Read the model definition and answer for the solid it produces. Units are mm, in the model's axes. Face numbers are marked on the shaded views. A direction names the side the tool comes from. Coordinates: 2 decimals unless noted, no trailing zeros. Loops run counter-clockwise (first coordinate to the right, second up) from the corner with the lowest first, then second, coordinate; pieces in that order, holes last. Notation, with made-up numbers: (-14.5, 32.5) - (-5.5, 32.5) arc R26 cw to (-5.5, 66.5) - close; hole circle Ø3 at (54.5, 12). An arc over 180 degrees is marked (long way). Use one line per item in the form item = value. Start each with the question number.
1) A cutting plane is placed at A-A (y = 12). Give the vertices of the cut face in (x, z).
2) Which of the six approach directions +Z, -Z, +X, -X, +Y, -Y give full straight-line access (tool end or side, diameter ignored) to the marked faces 1, 2, 3, 4 and 5?
3) A cutting plane is placed at C-C (x = -4). Give the vertices of the cut face in (y, z), and give its area (4 significant figures).
4) Consider line 1 (Y direction, x = -4, z = 2.05); line 2 (Z direction, x = -3.25, y = 8.25); line 3 (Z direction, x = -7, y = 3.5). Determine where each line is inside the solid, lowest interval first.
5) A cutting plane is placed at D-D (x = -6). Give the vertices of the cut face in (y, z).
6) Each of these flat-tipped pins is pushed along its axis until it touches: P1, Ø1.9, axis at x = -4, y = 12, coming from the +Z side; P2, Ø5.5, axis at y = 8.5, z = 29, coming from the -X side; P3, Ø5, axis at x = -4.5, z = 13.5, coming from the +Y side; P4, Ø4, axis at x = -5.5, y = 12, coming from the +Z side. Where does it stop, or does it pass through?
7) A cutting plane is placed at B-B (y = 10). Give the vertices of the cut face in (x, z), and give its area (3 significant figures).
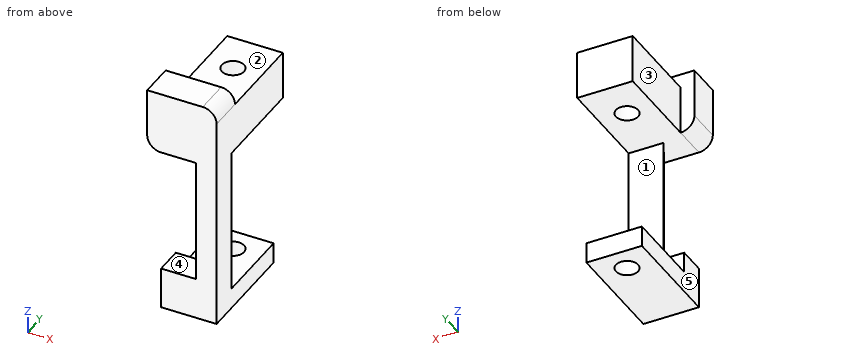
from build123d import *

# Parameters (mm, degrees)
BOSS_EXTRUDE1_DEPTH = 8
CUT_EXTRUDE2_DEPTH  = 21
BOSS_EXTRUDE2_DEPTH = 3
BOSS_EXTRUDE5_DEPTH = 5
SKETCH6_R           = 1.6
CUT_EXTRUDE3_DEPTH  = 38.215588132
SKETCH12_W          = 8
SKETCH12_H          = 3
CUT_EXTRUDE4_DEPTH  = 0.5


with BuildPart() as part:
    # Sketch1 → Boss-Extrude1 (new body)
    with BuildSketch(Plane(origin=(0, 0, 0), x_dir=(0, 0, -1), z_dir=(1, 0, 0))):
        Polygon((0, 0), (0, 16), (-3, 16), (-3, 4), (-24, 4), (-24, 18), (-31, 18), (-31, 0), align=None)
    extrude(amount=-BOSS_EXTRUDE1_DEPTH)

    # Sketch5 → Cut-Extrude2 (cut)
    with BuildSketch(Plane.XY.offset(3)):
        Polygon((-8, 0), (-3, 0), (-5, 4), (-8, 4), align=None)
    extrude(amount=CUT_EXTRUDE2_DEPTH, mode=Mode.SUBTRACT)

    # Sketch8 → Boss-Extrude2 (add)
    with BuildSketch(Plane.XY.offset(3)):
        Polygon((-8, 4), (-5, 4), (-3, 0), (-8, 0), align=None)
    extrude(amount=BOSS_EXTRUDE2_DEPTH)

    # Sketch11 → Boss-Extrude5 (add)
    with BuildSketch(Plane.XZ):
        with BuildLine():
            Line((-10, 26), (-10, 33))
            Line((-10, 33), (-2, 33))
            ThreePointArc((-2, 33), (-0.585786438, 32.414213562), (0, 31))
            Line((0, 31), (-8, 31))
            Line((-8, 31), (-8, 24))
            ThreePointArc((-8, 24), (-9.414213562, 24.585786438), (-10, 26))
        make_face()
    extrude(amount=-BOSS_EXTRUDE5_DEPTH)

    # Sketch6 → Cut-Extrude3 (cut, through all)
    with BuildSketch(Plane.XY.offset(31)):
        with Locations((-4, 12)):
            Circle(SKETCH6_R)
    extrude(amount=-CUT_EXTRUDE3_DEPTH, mode=Mode.SUBTRACT)

    # Sketch12 → Cut-Extrude4 (cut)
    with BuildSketch(Plane(origin=(0, 16, 0), x_dir=(1, 0, 0), z_dir=(0, 1, 0))):
        with Locations((-4, -1.5)):
            Rectangle(SKETCH12_W, SKETCH12_H)
    extrude(amount=-CUT_EXTRUDE4_DEPTH, mode=Mode.SUBTRACT)


solid = part.part
Found:
q1.outline = (-8, 0) - (-5.6, 0) - (-5.6, 3) - (-8, 3) - close; (-8, 24) - (-5.6, 24) - (-5.6, 31) - (-8, 31) - close; (-2.4, 0) - (0, 0) - (0, 3) - (-2.4, 3) - close; (-2.4, 24) - (0, 24) - (0, 31) - (-2.4, 31) - close
q2.face_1 = +X, -X, +Y
q2.face_2 = +Z, +X, -X, +Y
q2.face_3 = +Z, -Z, -X, +Y
q2.face_4 = -X, -Y
q2.face_5 = -Z, -X, +Y, -Y
q3.outline = (0, 0) - (10.4, 0) - (10.4, 3) - (4, 3) - (4, 24) - (10.4, 24) - (10.4, 31) - (5, 31) - (5, 33) - (0, 33) - (0, 24) - (2, 24) - (2, 6) - (0, 6) - close; (13.6, 0) - (15.5, 0) - (15.5, 3) - (13.6, 3) - close; (13.6, 24) - (18, 24) - (18, 31) - (13.6, 31) - close
q3.area = 198.5 mm^2
q4.line_1 = 0 to 10.4, 13.6 to 15.5
q4.line_2 = 0 to 3, 24 to 31
q4.line_3 = 0 to 6, 24 to 33
q5.outline = (0, 0) - (15.5, 0) - (15.5, 3) - (4, 3) - (4, 6) - (0, 6) - close; (0, 24) - (18, 24) - (18, 31) - (5, 31) - (5, 33) - (0, 33) - close
q6.P1 = through
q6.P2 = -8
q6.P3 = 4
q6.P4 = 31
q7.outline = (-8, 0) - (0, 0) - (0, 3) - (-8, 3) - close; (-8, 24) - (0, 24) - (0, 31) - (-8, 31) - close
q7.area = 80.0 mm^2
